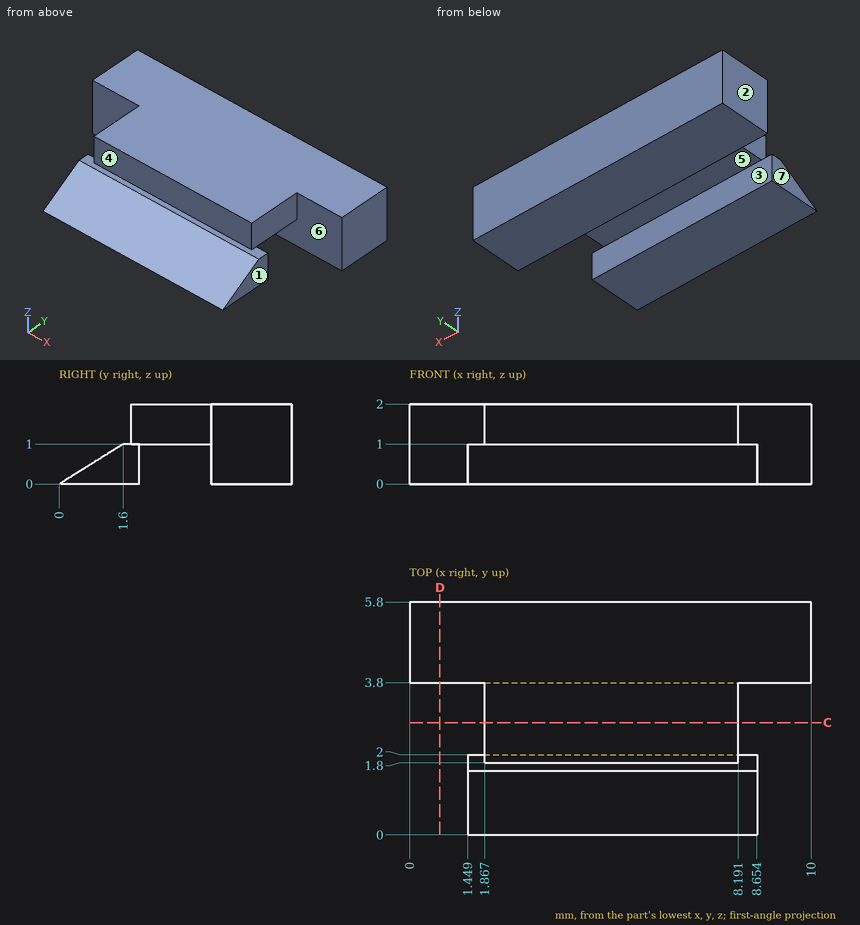
Source: three-view drawing plus pictorial views. Frame: mm from the lowest corner of the part. A direction names the side the tool comes from. Coordinates: 2 decimals unless noted, no trailing zeros. Order: outer loops, then holes, each group sorted by start corner. A loop starts at its lowest first (then second) coordinate and runs counter-clockwise, first axis right, second up.
Item 1: Cut plane D-D (x = 0.75). Return loops of the section in (y, z).
Output values:
outline: (3.8, 0) - (5.8, 0) - (5.8, 2) - (3.8, 2) - close
Item 2: Set-up query: the marked faces 1, 2 and 3. Return all of +Z, -Z, +X, -X, +Y, -Y with unobstructed straight access to the full face (end or side cutting, diameter ignored); none if empty.
Output values:
face 1: +Z, -Z, +X, -Y
face 2: +Z, -Z, -X, +Y, -Y
face 3: -Z, +X, -X
Item 3: First-contact query: P1, Ø1.1, axis at y = 1.5, z = 0.5, coming from the -X side; P2, Ø0.8, axis at x = 4.5, z = 1.5, coming from the -Y side; P3, Ø0.5, axis at x = 6.5, y = 3.5, coming from the -Z side. Flat tips, straight axial feed; report the tip coordinate or a pass-through.
Output values:
P1: stops at x = 1.45
P2: stops at y = 1.8
P3: stops at z = 1
Item 4: Material intervals for line 1 (Y direction, x = 3, z = 1.05); line 2 (Z direction, x = 6.5, y = 2.4); line 3 (Y direction, x = 1.75, z = 1.8), sorted ascending.
Output values:
line 1: y = 1.8 to 5.8
line 2: z = 1 to 2
line 3: y = 3.8 to 5.8
Item 5: Cut plane C-C (y = 2.8). Return loops of the section in (x, z).
Output values:
outline: (1.87, 1) - (8.19, 1) - (8.19, 2) - (1.87, 2) - close
Item 6: Pull-direction query (Y, two-part tool) for the marked faces 4, 5, 6 and 7; classes: pulls with the +Y half, pulls with the -Y half, needs draft (parallel to the pull), parting line crosses it, or undercut.
Output values:
face 4: pulls with the -Y half
face 5: undercut
face 6: undercut
face 7: needs draft
